from build123d import *

# Parameters (mm, degrees)
PAD002_DEPTH = 85
PAD001_DEPTH = 100
SKETCH_W     = 170
SKETCH_H     = 30
PAD_DEPTH    = 70
SKETCH003_R  = 15
PAD003_DEPTH = 20


with BuildPart() as pad002:
    # Sketch002 → Pad002 (new body)
    with BuildSketch(Plane.XZ):
        with BuildLine():
            Line((-48, 140), (-65, 140))
            Line((-65, 140), (-65, 55))
            Line((-65, 55), (65, 55))
            Line((65, 55), (65, 140))
            Line((65, 140), (48, 140))
            ThreePointArc((-48, 140), (0, 92), (48, 140))
        make_face()
    extrude(amount=PAD002_DEPTH)


with BuildPart() as pad001:
    # Sketch001 → Pad001 (new body)
    with BuildSketch(Plane.XZ):
        with BuildLine():
            Line((-85, 0), (-85, 30))
            Line((-85, 30), (85, 30))
            Line((85, 30), (85, 0))
            Line((85, 0), (110, 0))
            Line((110, 0), (110, 30))
            ThreePointArc((110, 30), (102.67767, 47.67767), (85, 55))
            Line((85, 55), (-85, 55))
            ThreePointArc((-85, 55), (-102.67767, 47.67767), (-110, 30))
            Line((-110, 30), (-110, 0))
            Line((-110, 0), (-85, 0))
        make_face()
    extrude(amount=PAD001_DEPTH)


with BuildPart() as pad:
    # Sketch → Pad (new body)
    with BuildSketch(Plane.XZ):
        with Locations((0, 15)):
            Rectangle(SKETCH_W, SKETCH_H)
    extrude(amount=PAD_DEPTH)


with BuildPart() as fusion:
    # Sketch003 → Pad003 (new body)
    with BuildSketch(Plane.XZ):
        with BuildLine():
            Line((65, 0), (145, 0))
            Line((145, 0), (145, 90))
            ThreePointArc((145, 90), (131.819805, 121.819805), (100, 135))
            Line((100, 135), (65, 135))
            Line((65, 135), (65, 0))
        make_face()
        with Locations((100, 90)):
            Circle(SKETCH003_R, mode=Mode.SUBTRACT)
        with BuildLine():
            Line((-65, 0), (-145, 0))
            Line((-145, 0), (-145, 90))
            ThreePointArc((-100, 135), (-131.819805, 121.819805), (-145, 90))
            Line((-100, 135), (-65, 135))
            Line((-65, 135), (-65, 0))
        make_face()
        with Locations((-100, 90)):
            Circle(SKETCH003_R, mode=Mode.SUBTRACT)
    extrude(amount=PAD003_DEPTH)

    # Fusion: union Pad002, Pad001, Pad
    add(pad002.part)
    add(pad001.part)
    add(pad.part)


solid = fusion.part
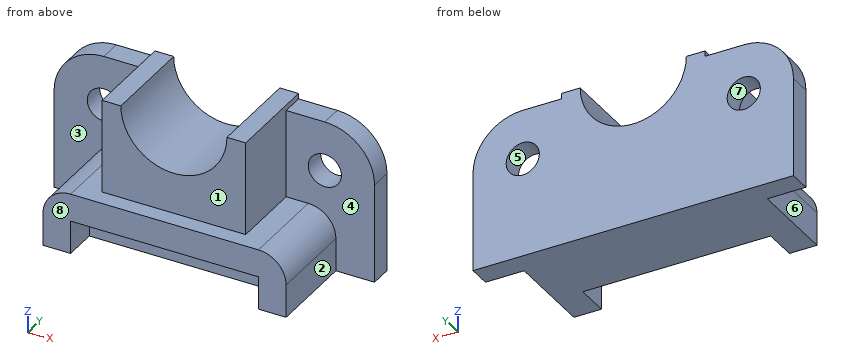
Read the model definition and answer for the solid it produces. Units are mm, in the model's axes. Face numbers are marked on the shaded views. A direction names the side the tool comes from. Round coordinates to 2 decimals unless told otherwise and drop trailing zeros. Write each loop counter-clockwise with the first axis right and the second up, starting at its lowest first coordinate (ties: lowest second). Pieces come first, ordered by that corner, then holes.
1. Straight lines are drawn through the part: L1, parallel to Z at x = 100, y = -11.5; L2, parallel to Y at x = -38, z = 24; L3, parallel to X at y = -18, z = 99. For each, find the intervals that lie inside material, in ascending order.
2. Given pin 1 Ø16 at (x, y) = (86.5, -10.5) entering from +Z; pin 2 Ø2 at (y, z) = (-25.5, 14.5) entering from -X; pin 3 Ø2 at (y, z) = (-45, 105) entering from +X, each flat-ended and moving along its own axis, determine where each tip first touches the part or whether it passes through.
3. The part is cut by section A-A, the plane y = -76. Determine the outline of the cut face in (x, z), then the cut area to 3 significant figures.
4. Determine the mould class of the marked faces 5, 6, 7 and 8 for opening direction X: pulls with the +X half, pulls with the -X half, needs draft (parallel to the pull), parting line crosses it, or undercut.
5. The part is cut by section B-B, the plane z = 11. Determine the outline of the cut face in (x, y), then the cut area to 3 significant figures.
6. The part is cut by section C-C, the plane x = 88.5. Determine the outline of the cut face in (y, z), then the cut area to 3 significant figures.
7. The part is cut by section D-D, the plane z = 129. Determine the outline of the cut face in (x, y), then the cut area to 3 significant figures.
8. Which of the six approach directions +Z, -Z, +X, -X, +Y, -Y give full straight-line access (tool end or side, diameter ignored) to the marked faces 1, 2, 3 and 4?
Values:
1. L1: z = 0 to 75, 105 to 135
1. L2: y = -70 to 0
1. L3: x = -144.09 to -112, -88 to -24.96, 24.96 to 88, 112 to 144.09
2. pin 1: stops at z = 135
2. pin 2: stops at x = -110
2. pin 3: stops at x = 65
3. outline: (-110, 0) - (-85, 0) - (-85, 30) - (85, 30) - (85, 0) - (110, 0) - (110, 30) arc R25 ccw to (85, 55) - (65, 55) - (65, 140) - (48, 140) arc R48 cw to (-48, 140) - (-65, 140) - (-65, 55) - (-85, 55) arc R25 ccw to (-110, 30) - close
3. area: 14,200 mm2
4. face 5: undercut
4. face 6: pulls with the -X half
4. face 7: undercut
4. face 8: needs draft
5. outline: (-145, -20) - (-110, -20) - (-110, -100) - (-85, -100) - (-85, -70) - (85, -70) - (85, -100) - (110, -100) - (110, -20) - (145, -20) - (145, 0) - (-145, 0) - close
5. area: 18,300 mm2
6. outline: (-100, 0) - (0, 0) - (0, 80.37) - (-20, 80.37) - (-20, 54.75) - (-100, 54.75) - close; (-20, 99.63) - (0, 99.63) - (0, 135) - (-20, 135) - close
6. area: 6,700 mm2
7. outline: (-122.45, -20) - (-65, -20) - (-65, -85) - (-46.72, -85) - (-46.72, 0) - (-122.45, 0) - close; (46.72, -85) - (65, -85) - (65, -20) - (122.45, -20) - (122.45, 0) - (46.72, 0) - close
7. area: 5,410 mm2
8. face 1: +Z, +X, -X, -Y
8. face 2: +Z, -Z, +X, -Y
8. face 3: +Z, -X, -Y
8. face 4: +Z, +X, -Y
